Design review of the part built by this model. Coordinates are the model's own, in mm. Coordinates: 2 decimals unless noted, no trailing zeros. Loops run counter-clockwise (first coordinate to the right, second up) from the corner with the lowest first, then second, coordinate; pieces in that order, holes last.
Q1. Wall thickness on probe 1 along X at (y, z) = (7.5, 1.25); probe 2 along Y at (x, z) = (-25.5, 1); probe 3 along Y at (x, z) = (6.5, 0.95): over which ranges is each line inside the solid? List them lowest first.
Q2. Add section C-C on x = 19. Give the boundary of the cut face in (y, z).
Q3. Add section B-B on z = 1.2. Give the number of separate pieces and of enclosed holes in the cut face, and give its area (3 significant figures).
Q4. Add section D-D on x = 31. Give the boundary of the cut face in (y, z), and give its area (3 significant figures).
Q5. Draft analysis for pull direction X (two halves, no side actions). For faces 1 (the face through (-1, 9, 0)), 2 (the face through (6.988, 60.673, 0.789)), 3 (the face through (-20.35, 51.64, 0.79)), 4 (the face through (-0.649, 64.997, 0.789)), state which applies: released by +X, released by -X, zero draft, split by the parting line, or undercut.
Q6. Add section A-A on x = 0. Give the boundary of the cut face in (y, z).
Q7. For P1, Ø3, axis at x = -7.06, y = 59.08, coming from the -Z side, flat-tipped, find the tip position at first contact; note if it passes through.
Autodesk Inventor part; units mm, degrees
ref_plane "YZ Plane" through (0, 0, 0) normal (1, 0, 0) x (0, 1, 0)
ref_plane "XZ Plane" through (0, 0, 0) normal (0, 1, 0) x (-1, 0, 0)
ref_plane "XY Plane" through (0, 0, 0) normal (0, 0, 1) x (1, 0, 0)
sketch "スケッチ1" plane through (0, 0, 0) normal (0, 0, 1) x (1, 0, 0)
  circle A0 centre (0, 0) radius 65 construction
  line L0 (-42.5, 65) -> (42.5, 65) construction
  line L1 (42.5, 65) -> (42.5, -65) construction
  line L2 (42.5, -65) -> (-42.5, -65) construction
  line L3 (-42.5, -65) -> (-42.5, 65) construction
  arc A1 (42.5, 49.1808) -> (-42.5, 49.1808) centre (0, 0) ccw
  line L4 (-42.5, 49.1808) -> (-42.5, -49.1808)
  line L5 (42.5, 49.1808) -> (42.5, -49.1808)
  arc A2 (-42.5, -49.1808) -> (42.5, -49.1808) centre (0, 0) ccw
  line L6 (42.5, -49) -> (-42.5, -49)
  point P0 (0, 65)
  dimension "d0" = 130
  dimension "d1" = 85
  dimension "d41" = 49
extrude "基板" add sketch "スケッチ1" along normal blind 1.6 contours L5 L6 L4 A1
sketch "スケッチ2" plane through (0, 0, 1.6) normal (0, 0, 1) x (1, 0, 0)
  line L0 (0, 110.7931) -> (0, -110.7931) construction
  line L1 (-42.5, 49.1808) -> (-42.5, -49) construction
  line L2 (-63.4163, -10) -> (63.4163, -10) construction
  point P0 (0, 0)
  point P1 (0, 0)
  point P2 (0, 0)
  point P3 (-42.5, -49.1808)
  point P4 (-25.5, -27.5)
  point P5 (-25.5, 7.5)
  point P6 (25.5, -27.5)
  point P7 (25.5, 7.5)
  point P8 (0, -10)
  dimension "d38" = 35
  dimension "d39" = 17
  dimension "d40" = 10
hole "モータ取付穴" at (-25.5, -27.5, 1.6) at (-25.5, 7.5, 1.6) at (25.5, -27.5, 1.6) at (25.5, 7.5, 1.6) direction (0, 0, -1) diameter 2.1 end through all
sketch "スケッチ3" plane through (0, 0, 1.6) normal (0, 0, 1) x (1, 0, 0)
  line L0 (0, 0) -> (0, 55.332) construction
  line L1 (-15.38, 55) -> (15.38, 55) construction
  line L2 (0, 46.85) -> (-7.0581, 50.925) construction
  line L3 (-7.0581, 50.925) -> (-7.0581, 59.075) construction
  line L4 (-7.0581, 59.075) -> (0, 63.15) construction
  line L5 (0, 63.15) -> (7.0581, 59.075) construction
  line L6 (7.0581, 59.075) -> (7.0581, 50.925) construction
  line L7 (7.0581, 50.925) -> (0, 46.85) construction
  arc A0 (42.5, 49.1808) -> (-42.5, 49.1808) centre (0, 0) ccw construction
  point P0 (0, 55)
  point P1 (0, 55)
  point P2 (0, 65)
  dimension "d17" = 16.3
  dimension "d18" = 10
hole "ボールキャスター取付穴" at (-7.0581, 59.075, 1.6) at (7.0581, 59.075, 1.6) at (0, 46.85, 1.6) direction (0, 0, -1) diameter 3.2 end through all
sketch "スケッチ5" plane through (0, 0, 1.6) normal (0, 0, 1) x (1, 0, 0)
  line L0 (0, 0) -> (0, 96.0936) construction
  line L1 (-67.6385, -10) -> (77.8935, -10) construction
  point P0 (-19, 52.5)
  point P1 (19, 52.5)
  dimension "d42" = 38
  dimension "d43" = 10
  dimension "d44" = 62.5
hole "穴4" at (-19, 52.5, 1.6) at (19, 52.5, 1.6) direction (0, 0, -1) diameter 3.2 end through all
properties part number "BaseBoard2"
Entries:
1. probe 1: x = -42.5 to -26.55, -24.45 to 24.45, 26.55 to 42.5
1. probe 2: y = -49 to -28.55, -26.45 to 6.45, 8.55 to 59.79
1. probe 3: y = -49 to 57.58, 60.57 to 64.67
2. outline: (-49, 0) - (50.9, 0) - (50.9, 1.6) - (-49, 1.6) - close; (54.1, 0) - (62.16, 0) - (62.16, 1.6) - (54.1, 1.6) - close
3. separate pieces: 1
3. enclosed holes: 9
3. area: 9,210 mm2
4. outline: (-49, 0) - (57.13, 0) - (57.13, 1.6) - (-49, 1.6) - close
4. area: 170 mm2
5. face 1: zero draft
5. face 2: undercut
5. face 3: undercut
5. face 4: split by the parting line
6. outline: (-49, 0) - (45.25, 0) - (45.25, 1.6) - (-49, 1.6) - close; (48.45, 0) - (65, 0) - (65, 1.6) - (48.45, 1.6) - close
7. P1: passes through
